Geometry check sheet. Reference: drawing and pictorial views, mm from the part's lowest x, y, z. A direction names the side the tool comes from. Round coordinates to 2 decimals unless told otherwise and drop trailing zeros. Write each loop counter-clockwise with the first axis right and the second up, starting at its lowest first coordinate (ties: lowest second). Pieces come first, ordered by that corner, then holes. Notation, with made-up numbers: M 72.25,87 L 106.25,87 A37 ccw 106.25,126 Z; hole C 72.25,44 d9. An arc over 180 degrees is marked long. One line per question, with ' | ' between items.
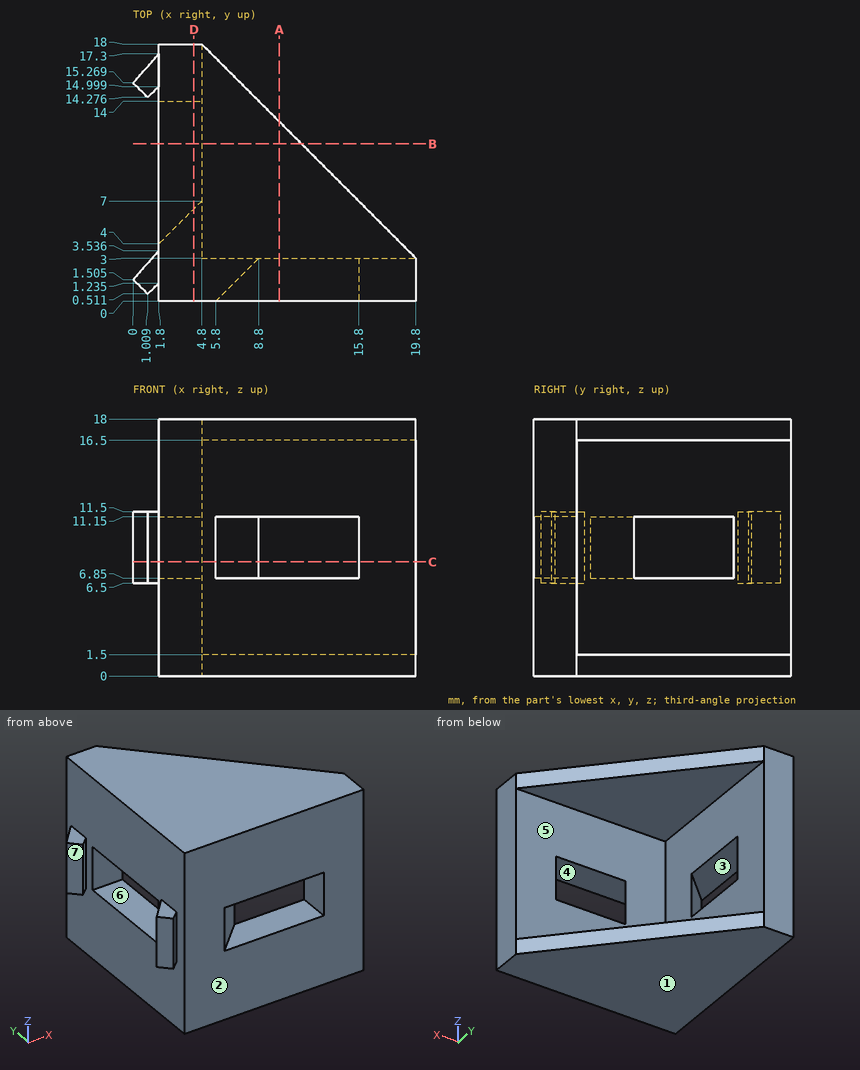
1. Mould release check, pull along Y, two halves, no side actions. Record for the marked faces 1, 2 and 3: pulls with the +Y half, pulls with the -Y half, needs draft (parallel to the pull), parting line crosses it, or undercut.
Results:
face 1: needs draft | face 2: pulls with the -Y half | face 3: undercut
2. Tool access check on the marked faces 4, 5, 6 and 7. Record the directions out of +Z, -Z, +X, -X, +Y, -Y that give a thin tool (end or side, any length) a straight path to the whole face; none if there is none.
Results:
face 4: -Y | face 5: +X, +Y | face 6: -X | face 7: +Z, -Z, -X
3. Section check C-C, the plane z = 8. Record the cut outline in (x, y) (1 decimal).
Results:
outline: M 0,1.5 L 1,0.5 L 1.8,1.2 L 1.8,0 L 5.8,0 L 8.8,3 L 4.8,3 L 4.8,7 L 1.8,4 L 1.8,3.5 Z; M 0,15.3 L 1,14.3 L 1.8,15 L 1.8,14 L 4.8,14 L 4.8,18 L 1.8,18 L 1.8,17.3 Z; M 15.8,0 L 19.8,0 L 19.8,3 L 15.8,3 Z
4. Section check D-D, the plane x = 4.25. Record the cut outline in (y, z).
Results:
outline: M 0,0 L 18,0 L 18,18 L 0,18 Z; hole M 6.45,6.85 L 14,6.85 L 14,11.15 L 6.45,11.15 Z
5. Section check A-A, the plane x = 10.25. Record the cut outline in (y, z).
Results:
outline: M 0,0 L 12.55,0 L 12.55,1.5 L 3,1.5 L 3,6.85 L 0,6.85 Z; M 0,11.15 L 3,11.15 L 3,16.5 L 12.55,16.5 L 12.55,18 L 0,18 Z
6. Section check B-B, the plane y = 11. Record the cut outline in (x, z).
Results:
outline: M 1.8,0 L 11.8,0 L 11.8,1.5 L 4.8,1.5 L 4.8,6.85 L 1.8,6.85 Z; M 1.8,11.15 L 4.8,11.15 L 4.8,16.5 L 11.8,16.5 L 11.8,18 L 1.8,18 Z
7. Thickness scan on line 1 (Z direction, x = 10.75, y = 7); line 2 (Z direction, x = 12, y = 2); line 3 (X direction, y = 14.5, z = 4). Record the ranges inside material, lowest first.
Results:
line 1: z = 0 to 1.5, 16.5 to 18 | line 2: z = 0 to 6.85, 11.15 to 18 | line 3: x = 1.8 to 4.8
8. Go/stop test with flat-tipped pins: P1, Ø10, axis at y = 12.5, z = 3.5, coming from the -X side; P2, Ø7.5, axis at y = 14, z = 7, coming from the +X side; P3, Ø0.5, axis at x = 1, y = 1.5, coming from the -Z side; P4, Ø5, axis at y = 4.5, z = 15.5, coming from the -X side. Record where each tip stops, or that it passes through.
Results:
P1: stops at x = 0 | P2: stops at x = 4.8 | P3: stops at z = 6.5 | P4: stops at x = 1.8
